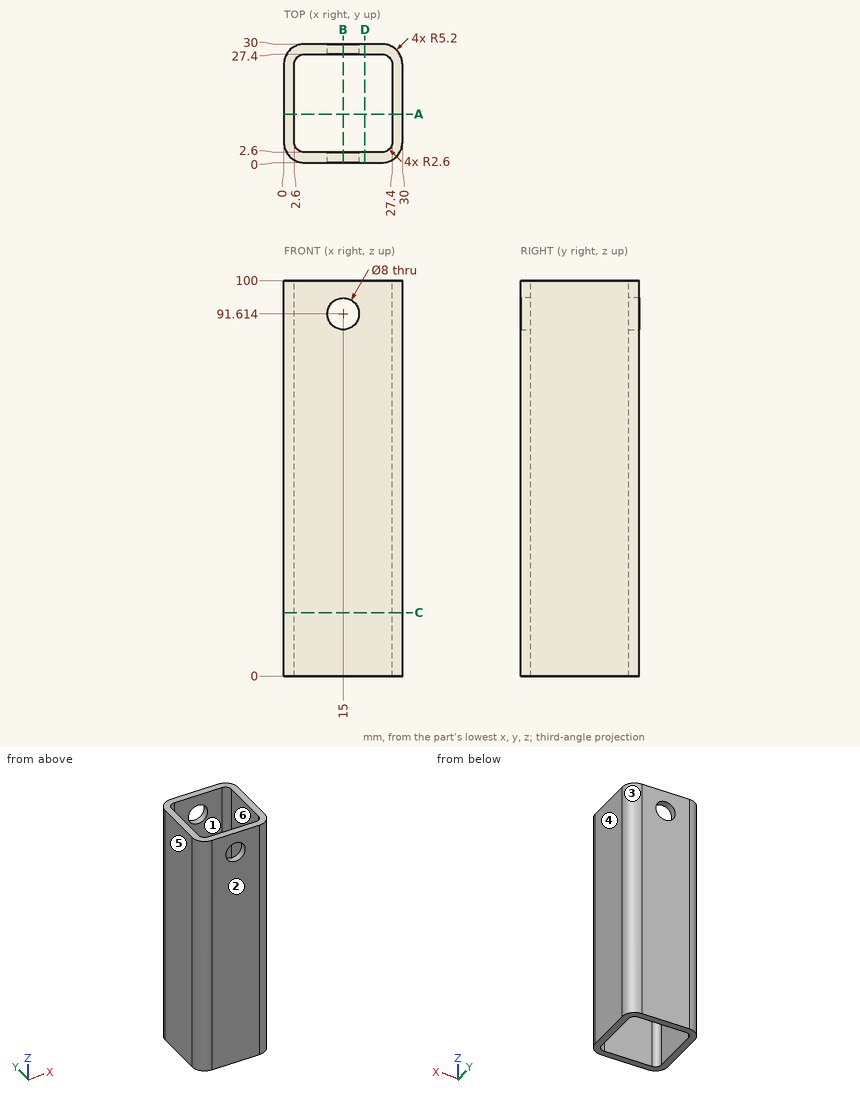
Can you work these out from the drawing? Everything is in mm from the part's minimum corner. A direction names the side the tool comes from. Round coordinates to 2 decimals unless told otherwise and drop trailing zeros. Order: outer loops, then holes, each group sorted by start corner. A loop starts at its lowest first (then second) coordinate and runs counter-clockwise, first axis right, second up.
(1) If we section it at C-C (z = 16): Please give me the cut outline in (x, y).
Results are:
outline: (0, 5.2) arc R5.2 ccw to (5.2, 0) - (24.8, 0) arc R5.2 ccw to (30, 5.2) - (30, 24.8) arc R5.2 ccw to (24.8, 30) - (5.2, 30) arc R5.2 ccw to (0, 24.8) - close; hole (2.6, 5.2) arc R2.6 ccw to (5.2, 2.6) - (24.8, 2.6) arc R2.6 ccw to (27.4, 5.2) - (27.4, 24.8) arc R2.6 ccw to (24.8, 27.4) - (5.2, 27.4) arc R2.6 ccw to (2.6, 24.8) - close
(2) If I drill on L1, parallel to X at y = 20, z = 38; L2, parallel to X at y = 26.75, z = 54, over which ranges is the centre line in solid material (lowest first)?
Results are:
L1: x = 0 to 2.6, 27.4 to 30
L2: x = 0.38 to 3.48, 26.52 to 29.62
(3) On a 3-axis mill with a long thin cutter (end or side, diameter ignored), from which of +Z, -Z, +X, -X, +Y, -Y can I reach the whole of each face in a straight line? I mean the marked faces 5 and 6. Say none if no direction works.
Results are:
face 5: +Z, -Z, -X, +Y, -Y
face 6: +Z, -Z
(4) We'd pull the mould along Y, two halves only. Please class the marked faces 1, 2, 3 and 4: +Y half, -Y half, draft (parallel to the pull), parting line (faces both ways), or undercut.
Results are:
face 1: undercut
face 2: -Y half
face 3: +Y half
face 4: draft
(5) If we section it at A-A (y = 12.25): Please give me the cut outline in (x, z).
Results are:
outline: (0, 0) - (2.6, 0) - (2.6, 100) - (0, 100) - close; (27.4, 0) - (30, 0) - (30, 100) - (27.4, 100) - close
(6) I'm going to push flat-ended pins straight in: pin 1 (6 mm diameter, centred on y = 9.5, z = 26, fed in from -X); pin 2 (3 mm diameter, centred on x = 20, y = 24, fed in from +Z). Where does each tip first touch, or does it pass through?
Results are:
pin 1: stops at x = 0
pin 2: passes through
(7) If we section it at B-B (x = 15): Please give me the cut outline in (y, z) (1 decimal).
Results are:
outline: (0, 0) - (2.6, 0) - (2.6, 87.6) - (0, 87.6) - close; (0, 95.6) - (2.6, 95.6) - (2.6, 100) - (0, 100) - close; (27.4, 0) - (30, 0) - (30, 87.6) - (27.4, 87.6) - close; (27.4, 95.6) - (30, 95.6) - (30, 100) - (27.4, 100) - close
